The listing builds one solid part. Answer for the finished solid, in the listing's coordinates (mm). Round coordinates to 2 decimals unless told otherwise and drop trailing zeros. Write each loop counter-clockwise with the first axis right and the second up, starting at its lowest first coordinate (ties: lowest second). Pieces come first, ordered by that corner, then holes. Notation, with made-up numbers: (-26, 71.25) -> (2, 71.25) arc R19 cw to (2, 102.25) -> close; hole circle Ø10 at (36, 15.25). An arc over 180 degrees is marked (long way). Write each question's results on one line, items separated by ' | '. Start each with the question number.
```python
from build123d import *

# Parameters (mm, degrees)
SKETCH1_W           = 35.56
SKETCH1_H           = 27.94
SKETCH1_R           = 1.267511842
SKETCH1_W_2         = 3.556
SKETCH1_H_2         = 13.97
SKETCH1_W_3         = 8.73125
SKETCH1_H_3         = 3.96875
SKETCH1_W_4         = 3.81
SKETCH1_H_4         = 8.128
SKETCH1_W_5         = 8.7379065
SKETCH1_H_5         = 6.35
BOSS_EXTRUDE1_DEPTH = 2.54
FILLET1_R           = 1.27


with BuildPart() as part:
    # Sketch1 → Boss-Extrude1 (new body)
    with BuildSketch(Plane.XY):
        with Locations((17.78, 13.97)):
            Rectangle(SKETCH1_W, SKETCH1_H)
        with Locations((2.54, 24.608738158)):
            Circle(SKETCH1_R, mode=Mode.SUBTRACT)
        with Locations(Location((25.24883074, 21.9075, 0), (0, 0, 180))):
            Circle(SKETCH1_R, mode=Mode.SUBTRACT)
        with Locations((9.34208074, 21.9075)):
            Circle(SKETCH1_R, mode=Mode.SUBTRACT)
        with Locations(Location((29.410568897, 24.608738158, 0), (0, 0, 180))):
            Circle(SKETCH1_R, mode=Mode.SUBTRACT)
        with Locations((25.52228569, 7.62)):
            Circle(SKETCH1_R, mode=Mode.SUBTRACT)
        with Locations((9.34208074, 7.62)):
            Circle(SKETCH1_R, mode=Mode.SUBTRACT)
        with Locations((2.54, 3.331261842)):
            Circle(SKETCH1_R, mode=Mode.SUBTRACT)
        with Locations((29.410568897, 3.331261842)):
            Circle(SKETCH1_R, mode=Mode.SUBTRACT)
        with Locations((32.47553569, 14.486722307)):
            Rectangle(SKETCH1_W_2, SKETCH1_H_2, mode=Mode.SUBTRACT)
        with Locations((16.50170574, 24.685625)):
            Rectangle(SKETCH1_W_3, SKETCH1_H_3, mode=Mode.SUBTRACT)
        with Locations((7.7109414, 13.97)):
            Rectangle(SKETCH1_W_4, SKETCH1_H_4, mode=Mode.SUBTRACT)
        with Locations((16.62537749, 4.445)):
            Rectangle(SKETCH1_W_5, SKETCH1_H_5, mode=Mode.SUBTRACT)
    extrude(amount=BOSS_EXTRUDE1_DEPTH)

    # Fillet1
    fillet1_edges = [part.edges().sort_by_distance(p)[0] for p in [
        (0, 27.94, 1.27),
        (35.56, 27.94, 1.27),
        (35.56, 0, 1.27),
        (0, 0, 1.27),
    ]]
    fillet(fillet1_edges, radius=FILLET1_R)


solid = part.part
```
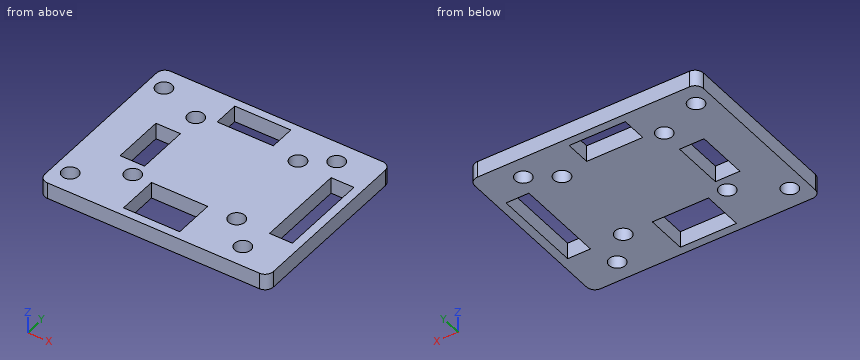
Q1. The part is cut by section A-A, the plane y = 19. Write down the section's boundary in (x, z).
Q2. The part is cut by section C-C, the plane z = 0.4. State how many separate pieces and enclosed holes the cut face has, then the cut area to 3 significant figures.
Q3. Each of these flat-tipped pins is pushed along its axis until it touches: pin 1 (3.5 mm diameter, centred on x = 29.41, y = 24.61, fed in from +Z); pin 2 (1.5 mm diameter, centred on x = 29.41, y = 3.33, fed in from -Z). Where does it stop, or does it pass through?
Q4. Find the intervals of material crossed by line 1 (X direction, y = 17.25, z = 2.1); line 2 (Y direction, x = 13, z = 1.9); line 3 (Y direction, x = 2.54, z = 1.35), in increasing order.
Q5. The part is cut by section B-B, the plane x = 2.54. Write down the section's boundary in (y, z).
Q6. The part is cut by section D-D, the plane y = 25.5. Write down the section's boundary in (x, z).
Answers follow:
1) outline: (0, 0) -> (30.7, 0) -> (30.7, 2.54) -> (0, 2.54) -> close; (34.25, 0) -> (35.56, 0) -> (35.56, 2.54) -> (34.25, 2.54) -> close
2) separate pieces: 1 | enclosed holes: 12 | area: 781 mm^2
3) pin 1: z = 2.54 | pin 2: through
4) line 1: 0 to 5.81, 9.62 to 30.7, 34.25 to 35.56 | line 2: 0 to 1.27, 7.62 to 22.7, 26.67 to 27.94 | line 3: 0 to 2.06, 4.6 to 23.34, 25.88 to 27.94
5) outline: (0, 0) -> (2.06, 0) -> (2.06, 2.54) -> (0, 2.54) -> close; (4.6, 0) -> (23.34, 0) -> (23.34, 2.54) -> (4.6, 2.54) -> close; (25.88, 0) -> (27.94, 0) -> (27.94, 2.54) -> (25.88, 2.54) -> close
6) outline: (0, 0) -> (1.64, 0) -> (1.64, 2.54) -> (0, 2.54) -> close; (3.44, 0) -> (12.14, 0) -> (12.14, 2.54) -> (3.44, 2.54) -> close; (20.87, 0) -> (28.51, 0) -> (28.51, 2.54) -> (20.87, 2.54) -> close; (30.31, 0) -> (35.56, 0) -> (35.56, 2.54) -> (30.31, 2.54) -> close
